Can you work these out from the model? Positions are in its coordinate system, mm. Face numbers are marked on the shaded views. A direction names the side the tool comes from. Round coordinates to 2 decimals unless told otherwise and drop trailing zeros. Order: outer loops, then holes, each group sorted by start corner. A loop starts at its lowest first (then second) coordinate and runs counter-clockwise, first axis right, second up. Notation, with made-up numbers: (83, 65.5) -> (96, 65.5) arc R10 cw to (96, 82.5) -> close; hole circle Ø3 at (7.5, -16.5). An arc over 180 degrees is marked (long way). Use a Markdown table: item, result. Add a question column.
Q1. If we section it at C-C on x = -10: List the corners of the cut face in (y, z) for me, plus the area to 3 significant figures.
Q2. I need wall thicknesses on line 1 along X through (y, z) = (9.5, -6); line 2 along Z through (x, y) = (-15.5, 5.7); line 3 along Z through (x, y) = (-43, 9). Which ranges of each line are inside material? Lowest first, please. Write a range as [from, to].
Q3. If we section it at A-A on z = -4: List the corners of the cut face in (x, y) for me.
Q4. If we section it at B-B on y = 5.9: List the corners of the cut face in (x, z) for me.
Q5. We'd pull the mould along Z, two halves only. Please class the marked faces 1, 2, 3 and 4: +Z half, -Z half, draft (parallel to the pull), parting line (faces both ways), or undercut.
Q6. I'm going to push flat-ended pins straight in: pin 1 Ø1 at (x, y) = (-16.5, 9) entering from -Z; pin 2 Ø1 at (x, y) = (10.5, 8) entering from -Z; pin 3 Ø6 at (x, z) = (4, -7) entering from -Y; pin 4 Ø5.5 at (x, z) = (-11.08, -5.49) entering from +Y. Where does each tip first touch, or does it pass through?
Q7. If we section it at D-D on z = -7.75: List the corners of the cut face in (x, y) for me, plus the area to 3 significant figures.
Q8. For the marked faces 5 and 6, which set-ups out of +Z, -Z, +X, -X, +Y, -Y let a thin tool reach every point of the face, with its end or its side?
```python
from build123d import *

# Parameters (mm, degrees)
BOSS_EXTRUDE1_DEPTH = 15
F_20_0MM_1_D        = 20
SCALE_1_SCALE       = 0.3


with BuildPart() as part:
    # Sketch1 → Boss-Extrude1 (new body)
    with BuildSketch(Plane(origin=(0, 0, 0), x_dir=(1, 0, 0), z_dir=(0, 1, 0))):
        with BuildLine():
            Line((0, 20), (-100, 20))
            ThreePointArc((-100, 20), (-120, 0), (-100, -20))
            Line((-100, -20), (0, -20))
            ThreePointArc((0, -20), (20, 0), (0, 20))
        make_face()
        with BuildLine():
            ThreePointArc((0, 20), (12.75180627, 15.407512352), (19.64736126, 3.739143686))
            Line((19.64736126, 3.739143686), (70.3513219, 22.193876119))
            Line((70.3513219, 22.193876119), (76.50768448, 5.279408944))
            Line((76.50768448, 5.279408944), (100, 13.829912528))
            Line((100, 13.829912528), (89.7393957, 42.020691151))
            Line((89.7393957, 42.020691151), (70.04324064, 45.493654704))
            Line((70.04324064, 45.493654704), (0, 20))
        make_face()
    extrude(amount=BOSS_EXTRUDE1_DEPTH)

    # Ø20.0mm 맞춤핀 구멍1 (through all)
    with Locations(Plane(origin=(0, 15, 0), x_dir=(1, 0, 0), z_dir=(0, 1, 0))):
        with Locations((-100, 0), (0, 0)):
            Hole(F_20_0MM_1_D / 2)


with BuildPart() as part_1:
    # 축척1: scaled about (-15.835607979, 7.5, -7.836280523)
    add(part.part.scale(SCALE_1_SCALE).moved(Location((-11.084925585, 5.25, -5.485396366))))


solid = part_1.part
```
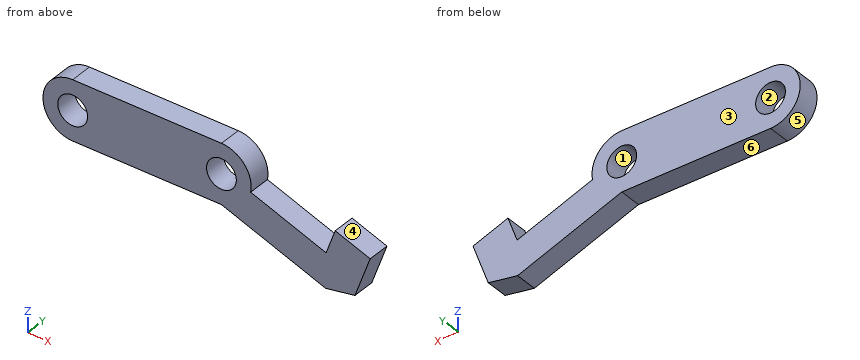
Answer below:
| question | item | result |
|---|---|---|
| 1 | outline | (5.25, -11.88) -> (9.75, -11.88) -> (9.75, -8.28) -> (5.25, -8.28) -> close; (5.25, -2.69) -> (9.75, -2.69) -> (9.75, 0.42) -> (5.25, 0.42) -> close |
| 1 | area | 30.2 mm² |
| 2 | line 1 | [-47.06, -44.04], [-38.13, -14.04], [-8.13, -5.11] |
| 2 | line 2 | [-11.49, 0.51] |
| 2 | line 3 | [-11.17, -7.79], [-3.18, 0.2] |
| 3 | outline | (-46.9, 5.25) -> (-43.69, 5.25) -> (-43.69, 9.75) -> (-46.9, 9.75) -> close; (-38.48, 5.25) -> (-13.69, 5.25) -> (-13.69, 9.75) -> (-38.48, 9.75) -> close; (-8.48, 5.25) -> (-5.27, 5.25) -> (-5.27, 9.75) -> (-8.48, 9.75) -> close |
| 4 | outline | (-41.08, -11.49) -> (-11.08, -11.49) -> (9.93, -19.13) -> (15.84, -18.09) -> (18.92, -9.63) -> (11.87, -7.07) -> (10.02, -12.14) -> (-5.19, -6.61) arc R6 ccw to (-11.08, 0.51) -> (-41.08, 0.51) arc R6 ccw to start; hole circle Ø6 at (-41.08, -5.49); hole circle Ø6 at (-11.08, -5.49) |
| 5 | face 1 | undercut |
| 5 | face 2 | undercut |
| 5 | face 3 | draft |
| 5 | face 4 | +Z half |
| 6 | pin 1 | z = -11.49 |
| 6 | pin 2 | z = -19.12 |
| 6 | pin 3 | y = 5.25 |
| 6 | pin 4 | through |
| 7 | outline | (-46.64, 5.25) -> (-43.05, 5.25) -> (-43.05, 9.75) -> (-46.64, 9.75) -> close; (-39.12, 5.25) -> (-13.05, 5.25) -> (-13.05, 9.75) -> (-39.12, 9.75) -> close; (-9.12, 5.25) -> (-2.05, 5.25) -> (-2.05, 9.75) -> (-9.12, 9.75) -> close; (11.62, 5.25) -> (13.74, 5.25) -> (13.74, 9.75) -> (11.62, 9.75) -> close |
| 7 | area | 175 mm² |
| 8 | face 5 | -X, +Y, -Y |
| 8 | face 6 | -Z, -X, +Y, -Y |
